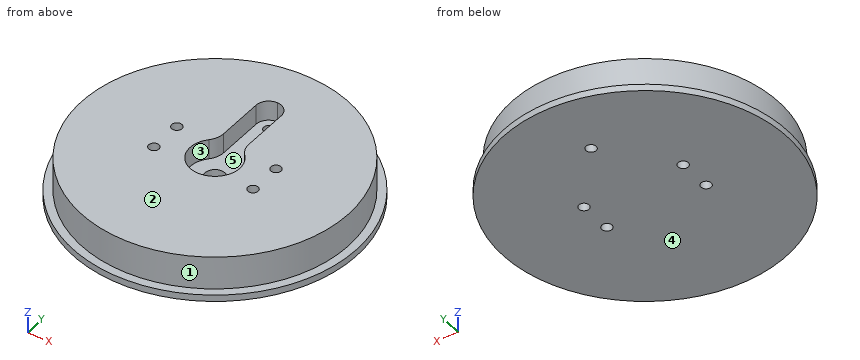
```python
from build123d import *

# Parameters (mm, degrees)
SKETCH_R        = 42.75
PAD_DEPTH       = 2
SKETCH001_R     = 40.25
PAD001_DEPTH    = 10
SKETCH002_R     = 7.5
POCKET_DEPTH    = 6
SKETCH003_W     = 7.6
SKETCH003_H     = 27.2
POCKET001_DEPTH = 6
FILLET_R        = 6
FILLET001_R     = 3.7999
SKETCH004_R     = 1.55
POCKET002_DEPTH = 6
SKETCH005_R     = 3
POCKET003_DEPTH = 3
SKETCH006_R     = 1.55
POCKET004_DEPTH = 12


with BuildPart() as part:
    # Sketch → Pad (new body)
    with BuildSketch(Plane.XY):
        Circle(SKETCH_R)
    extrude(amount=PAD_DEPTH)

    # Sketch001 (on Face3 of Pad) → Pad001 (join)
    with BuildSketch(Plane.XY.offset(2)):
        Circle(SKETCH001_R)
    extrude(amount=PAD001_DEPTH)

    # Sketch002 (on Face5 of Pad001) → Pocket (cut)
    with BuildSketch(Plane.XY.offset(12)):
        Circle(SKETCH002_R)
    extrude(amount=-POCKET_DEPTH, mode=Mode.SUBTRACT)

    # Sketch003 (on Face5 of Pocket) → Pocket001 (cut)
    with BuildSketch(Plane.XY.offset(12)):
        with Locations((0, 13.6)):
            Rectangle(SKETCH003_W, SKETCH003_H)
    extrude(amount=-POCKET001_DEPTH, mode=Mode.SUBTRACT)

    # Fillet
    fillet_edges = [part.edges().sort_by_distance(p)[0] for p in [
        (-3.8, 6.466065, 9),
        (3.8, 6.466065, 9),
    ]]
    fillet(fillet_edges, radius=FILLET_R)

    # Fillet001
    fillet001_edges = [part.edges().sort_by_distance(p)[0] for p in [
        (3.8, 27.2, 9),
        (-3.8, 27.2, 9),
    ]]
    fillet(fillet001_edges, radius=FILLET001_R)

    # Sketch004 (on Face12 of Fillet001) → Pocket002 (cut)
    with BuildSketch(Plane.XY.offset(6)):
        with Locations((0, 23.5)):
            Circle(SKETCH004_R)
    extrude(amount=-POCKET002_DEPTH, mode=Mode.SUBTRACT)

    # Sketch005 (on Face13 of Pocket002) → Pocket003 (cut)
    with BuildSketch(Plane.XY.offset(6)):
        Circle(SKETCH005_R)
    extrude(amount=-POCKET003_DEPTH, mode=Mode.SUBTRACT)

    # Sketch006 (on Face1 of Pocket003) → Pocket004 (cut)
    with BuildSketch(Plane.XY.offset(12)):
        with Locations((-15, 5)):
            Circle(SKETCH006_R)
        with Locations((15, 5)):
            Circle(SKETCH006_R)
        with Locations((15, -5)):
            Circle(SKETCH006_R)
        with Locations((-15, -5)):
            Circle(SKETCH006_R)
    extrude(amount=-POCKET004_DEPTH, mode=Mode.SUBTRACT)


solid = part.part
```
Design review of the part built by this model. Coordinates are the model's own, in mm. Face numbers are marked on the shaded views. A direction names the side the tool comes from. Give positions to 0.01 mm unless a question says otherwise; leave off trailing zeros. Write each loop counter-clockwise with the first axis right and the second up, starting at its lowest first coordinate (ties: lowest second). Pieces come first, ordered by that corner, then holes. Notation, with made-up numbers: (-39, 44.5) - (-6, 44.5) arc R16 cw to (-6, 54.5) - close; hole circle Ø4 at (-10, 24). An arc over 180 degrees is marked (long way). Return JSON: item names as keys, results as strings. Group by question number.
(1) We need section C-C, the plane y = 0. Give the boundary of the cut face in (x, z).
(2) To check wall thickness, follow probe 1 along Y at (x, z) = (15, 9); probe 2 along Z at (x, y) = (-17.5, 37); probe 3 along Z at (x, y) = (7, 2). State the ranges of each line that lie inside material, in increasing order.
(3) We need section A-A, the plane z = 8.5. Give the number of separate pieces and of enclosed holes in the cut face, then the cut area to 3 significant figures.
(4) Insertion check: pin 1 (3 mm diameter, centred on y = 13.5, z = 10.5, fed in from +X); pin 2 (1.5 mm diameter, centred on x = 29.5, z = 3.5, fed in from +Y); pin 3 (1.8 mm diameter, centred on x = 0.5, y = 0, fed in from +Z). Each pin has a flat end and moves straight along its axis. Give the tip position at first contact, or say it passes through.
(5) Mouldability with a two-part tool opening along X and no side actions: class the marked faces 1, 2 and 3 as +X half, -X half, draft (parallel to the pull), parting line (faces both ways), or undercut.
(6) Machinability: for the marked faces 4 and 5, which of the approach directions +Z, -Z, +X, -X, +Y, -Y give a long, thin tool a straight path to every point of the face, cutting with its end or side? Answer none if there is none.
(7) We need section D-D, the plane y = -32. Give the boundary of the cut face in (x, z).
(8) We need section B-B, the plane x = -15. Give the boundary of the cut face in (y, z), then the cut area to 3 significant figures.
Reported:
{
 "1": {"outline": "(-42.75, 0) - (42.75, 0) - (42.75, 2) - (40.25, 2) - (40.25, 12) - (7.5, 12) - (7.5, 6) - (3, 6) - (3, 3) - (-3, 3) - (-3, 6) - (-7.5, 6) - (-7.5, 12) - (-40.25, 12) - (-40.25, 2) - (-42.75, 2) - close"},
 "2": {"probe 1": "y = -37.35 to -6.55, -3.45 to 3.45, 6.55 to 37.35", "probe 2": "z = 0 to 2", "probe 3": "z = 0 to 6"},
 "3": {"separate pieces": "1", "enclosed holes": "5", "area": "4,730 mm2"},
 "4": {"pin 1": "stops at x = 38.42", "pin 2": "stops at y = 28.17", "pin 3": "stops at z = 3"},
 "5": {"face 1": "parting line", "face 2": "draft", "face 3": "undercut"},
 "6": {"face 4": "-Z, +X, -X, +Y, -Y", "face 5": "+Z"},
 "7": {"outline": "(-28.35, 0) - (28.35, 0) - (28.35, 2) - (24.41, 2) - (24.41, 12) - (-24.41, 12) - (-24.41, 2) - (-28.35, 2) - close"},
 "8": {"outline": "(-40.03, 0) - (-6.55, 0) - (-6.55, 12) - (-37.35, 12) - (-37.35, 2) - (-40.03, 2) - close; (-3.45, 0) - (3.45, 0) - (3.45, 12) - (-3.45, 12) - close; (6.55, 0) - (40.03, 0) - (40.03, 2) - (37.35, 2) - (37.35, 12) - (6.55, 12) - close", "area": "833 mm2"}
}
